Here's how the part is built. I have some questions about the finished solid (model axes, mm). Face numbers are marked on the shaded views. A direction names the side the tool comes from. Give positions to 0.01 mm unless a question says otherwise; leave off trailing zeros. Write each loop counter-clockwise with the first axis right and the second up, starting at its lowest first coordinate (ties: lowest second). Pieces come first, ordered by that corner, then holes. Notation, with made-up numbers: (79, -10.75) -> (106, -10.75) arc R23 cw to (106, 26.25) -> close; hole circle Ø10 at (-25.5, -18). An arc over 180 degrees is marked (long way). Use one line per item in the form item = value.
Autodesk Inventor part; units mm, degrees
ref_plane "YZ Plane" through (0, 0, 0) normal (1, 0, 0) x (0, 1, 0)
ref_plane "XZ Plane" through (0, 0, 0) normal (0, 1, 0) x (-1, 0, 0)
ref_plane "XY Plane" through (0, 0, 0) normal (0, 0, 1) x (1, 0, 0)
sketch "Эскиз1" plane through (0, 0, 0) normal (0, 0, 1) x (1, 0, 0)
  line L0 (0, 0) -> (0, 24) construction
  line L1 (0, 24) -> (4, 24) construction
  line L2 (4, 24) -> (4, 0)
  line L3 (4, 24) -> (7.5, 24)
  line L4 (7.5, 24) -> (7.5, 20.75)
  line L5 (7.5, 20.75) -> (6.5, 20.75)
  line L6 (6.5, 20.75) -> (6.5, 19.65)
  line L7 (6.5, 19.65) -> (7.5, 19.65)
  line L8 (7.5, 19.65) -> (7.5, 4.35)
  line L9 (7.5, 4.35) -> (6.5, 4.35)
  line L10 (6.5, 4.35) -> (6.5, 3.25)
  line L11 (6.5, 3.25) -> (7.5, 3.25)
  line L12 (7.5, 3.25) -> (7.5, 0)
  line L13 (7.5, 0) -> (4, 0)
  dimension "d0" = 24
  dimension "d1" = 4
  dimension "d3" = 3.5
  dimension "d4" = 3.25
  dimension "d5" = 1
  dimension "d6" = 1.1
  dimension "d7" = 15.3
  dimension "d8" = 1
  dimension "d9" = 1.1
revolve "Вращение1" add sketch "Эскиз1" angle 360 about axis through (0, 0, 0) along (0, 1, 0)
chamfer "Фаска1" distance 0.3 angle 45 2 edges at (-7.5, 24, 0) (-7.5, 0, 0)
sketch "Эскиз2" plane through (0, 24, 0) normal (0, 1, 0) x (1, 0, 0)
  circle A0 centre (0, 0) radius 4
  circle A1 centre (0, 0) radius 7.2
  circle A2 centre (0, 0) radius 6.5
  dimension "d14" = 13
extrude "Выдавливание1" cut sketch "Эскиз2" against normal blind 2 contours A2
chamfer "Фаска2" distance 0.3 angle 45 1 edges at (-6.5, 24, 0)
sketch "Эскиз4" plane through (0, 0, 0) normal (0, -1, 0) x (1, 0, 0)
  circle A0 centre (0, 0) radius 4
  circle A1 centre (0, 0) radius 7.2
  circle A2 centre (0, 0) radius 6.5
  dimension "d27" = 13
extrude "Выдавливание3" cut sketch "Эскиз4" against normal blind 2 contours A2
chamfer "Фаска4" distance 0.3 angle 45 1 edges at (-6.5, 0, 0)
properties part number "bearing"
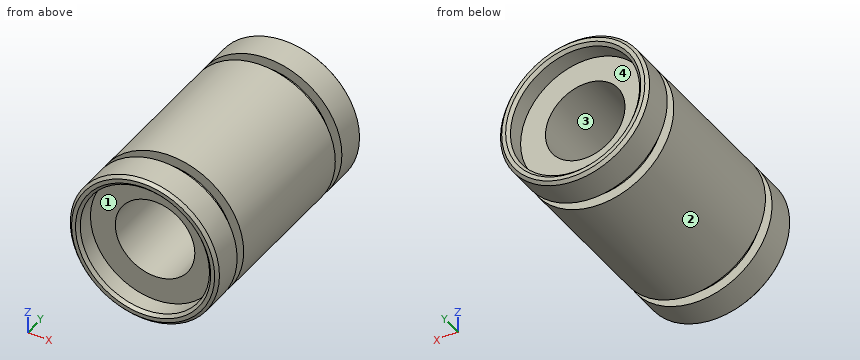
Q1. I want a section at A-A, the plane y = 15. Write out the boundary of the cut face in (x, z).
Result set:
outline = circle Ø15 at (0, 0); hole circle Ø8 at (0, 0)
Q2. Will these pins go through, and if not, where does the flat tip stop? pin 1 Ø6 at (y, z) = (19, 4) entering from -X; pin 2 Ø7.5 at (x, z) = (-1.5, 0.5) entering from -Y; pin 3 Ø1 at (y, z) = (4, -0.5) entering from +X.
Result set:
pin_1 = -7.43
pin_2 = 2
pin_3 = 7.5
Q3. If I drill on line 1 along Y through (x, z) = (2, -6.5); line 2 along X through (y, z) = (12.5, 0); line 3 along Z through (x, y) = (0, 22.25), over which ranges is the centre line in solid material (lowest first)? Write a range as from..to.
Result set:
line_1 = 0..3.25, 4.35..19.65, 20.75..24
line_2 = -7.5..-4, 4..7.5
line_3 = -7.5..-6.5, 6.5..7.5
Q4. If we mould it in two halves opening along X, with no side actions, what happens to the marked faces 1 and 2? For each: +X half, -X half, draft (parallel to the pull), parting line (faces both ways), or undercut.
Result set:
face_1 = undercut
face_2 = parting line
Q5. Which directions (+Z, -Z, +X, -X, +Y, -Y) give clear straight access to the entire face, cutting with the end or side of a thin tool? Please do the marked faces 3 and 4.
Result set:
face_3 = +Y, -Y
face_4 = +Y
